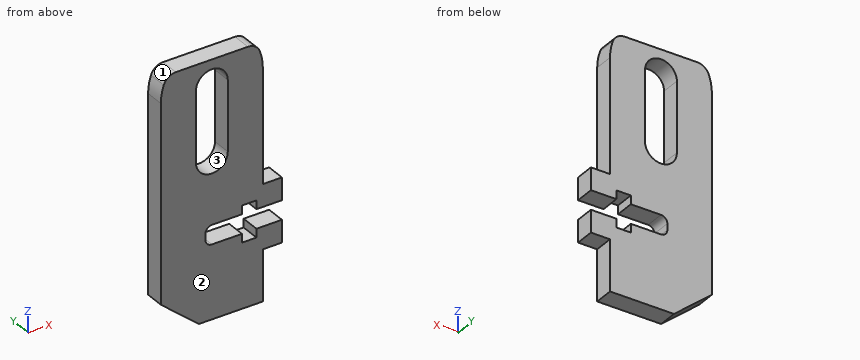
```python
from build123d import *

# Parameters (mm, degrees)
BOSS_EXTRUDE1_DEPTH     = 1.5
CUT_EXTRUDE1_DEPTH      = 38.54894195
CUT_EXTRUDE1_DEPTH_BACK = 38.54894195


with BuildPart() as part:
    # Sketch2 → Boss-Extrude1 (new, symmetric)
    with BuildSketch(Plane(origin=(0, 0, 0), x_dir=(1, 0, 0), z_dir=(0, 1, 0))):
        with BuildLine():
            Line((-8, 10.748624987), (-8, 30.870225))
            Line((-8, 30.870225), (-2.041232037, 35.870225))
            Line((-2.041232037, 35.870225), (8, 35.870225))
            Line((8, 35.870225), (8, 30.870225))
            Line((8, 30.870225), (8, 27.870225))
            Line((8, 27.870225), (11, 27.870225))
            Line((11, 27.870225), (11, 17.870225))
            Line((11, 17.870225), (8, 17.870225))
            Line((8, 17.870225), (8, 14.870225))
            Line((8, 14.870225), (8, 10.748624987))
            Line((8, 10.748624987), (8, 0))
            ThreePointArc((8, 0), (7.884788477, -1.35281583), (7.542472333, -2.666666667))
            ThreePointArc((7.542472333, -2.666666667), (6.811554788, -3.632993162), (5.656854249, -4))
            Line((5.656854249, -4), (-5.656854249, -4))
            ThreePointArc((-5.656854249, -4), (-6.811554788, -3.632993162), (-7.542472333, -2.666666667))
            ThreePointArc((-7.542472333, -2.666666667), (-7.884788477, -1.35281583), (-8, 0))
            Line((-8, 0), (-8, 10.748624987))
        make_face()
        with BuildLine():
            Line((-2.5, 0), (-2.5, 11))
            ThreePointArc((-2.5, 11), (0, 13.5), (2.5, 11))
            Line((2.5, 11), (2.5, 0))
            ThreePointArc((2.5, 0), (0, -2.5), (-2.5, 0))
        make_face(mode=Mode.SUBTRACT)
    extrude(amount=BOSS_EXTRUDE1_DEPTH, both=True)

    # Sketch4 → Cut-Extrude1 (cut, two sides: drawn at the far end of the back side and taken through both)
    with BuildSketch(Plane(origin=(0, 0, 0), x_dir=(1, 0, 0), z_dir=(0, 1, 0)).offset(-CUT_EXTRUDE1_DEPTH_BACK)):
        with BuildLine():
            Line((11, 24.370225), (7, 24.370225))
            Line((7, 24.370225), (7, 25.720225))
            Line((7, 25.720225), (4.73, 25.720225))
            Line((4.73, 25.720225), (4.73, 24.370225))
            Line((4.73, 24.370225), (0, 24.370225))
            ThreePointArc((0, 24.370225), (-0.707106781, 24.077331781), (-1, 23.370225))
            Line((-1, 23.370225), (-1, 22.370225))
            ThreePointArc((-1, 22.370225), (-0.707106781, 21.663118219), (0, 21.370225))
            Line((0, 21.370225), (4.73, 21.370225))
            Line((4.73, 21.370225), (4.73, 20.020225))
            Line((4.73, 20.020225), (7, 20.020225))
            Line((7, 20.020225), (7, 21.370225))
            Line((7, 21.370225), (11, 21.370225))
            Line((11, 21.370225), (11, 24.370225))
        make_face()
    extrude(amount=CUT_EXTRUDE1_DEPTH + CUT_EXTRUDE1_DEPTH_BACK, mode=Mode.SUBTRACT)


solid = part.part
```
The listing builds one solid part. Answer for the finished solid, in the listing's coordinates (mm). Face numbers are marked on the shaded views. Give positions to 0.01 mm unless a question says otherwise; leave off trailing zeros. Order: outer loops, then holes, each group sorted by start corner. A loop starts at its lowest first (then second) coordinate and runs counter-clockwise, first axis right, second up.
Item 1: Given pin 1 Ø1.5 at (x, y) = (9.5, -0.5) entering from +Z; pin 2 Ø0.9 at (y, z) = (0.5, -5) entering from +X; pin 3 Ø0.5 at (y, z) = (0.5, -23) entering from +X, each flat-ended and moving along its own axis, determine where each tip first touches the part or whether it passes through.
From the geometry:
pin 1: stops at z = -17.87
pin 2: stops at x = 8
pin 3: stops at x = -1
Item 2: Find the intervals of material crossed by probe 1 along X at (y, z) = (0.95, -11); probe 2 along Z at (x, y) = (5, -1.4); probe 3 along Z at (x, y) = (4.25, -0.95), in increasing order.
From the geometry:
probe 1: x = -8 to -2.5, 2.5 to 8
probe 2: z = -35.87 to -25.72, -20.02 to 4
probe 3: z = -35.87 to -24.37, -21.37 to 4
Item 3: The part is cut by section A-A, the plane x = 9.5. Give the vertices of the cut face in (y, z).
From the geometry:
outline: (-1.5, -27.87) - (1.5, -27.87) - (1.5, -24.37) - (-1.5, -24.37) - close; (-1.5, -21.37) - (1.5, -21.37) - (1.5, -17.87) - (-1.5, -17.87) - close
Item 4: The part is cut by section D-D, the plane x = 1.5. Give the vertices of the cut face in (y, z), and give its area (3 significant figures).
From the geometry:
outline: (-1.5, -35.87) - (1.5, -35.87) - (1.5, -24.37) - (-1.5, -24.37) - close; (-1.5, -21.37) - (1.5, -21.37) - (1.5, -13) - (-1.5, -13) - close; (-1.5, 2) - (1.5, 2) - (1.5, 4) - (-1.5, 4) - close
area: 65.6 mm2
Item 5: The part is cut by section B-B, the plane z = -4. Give the vertices of the cut face in (x, y), and give its area (3 significant figures).
From the geometry:
outline: (-8, -1.5) - (-2.5, -1.5) - (-2.5, 1.5) - (-8, 1.5) - close; (2.5, -1.5) - (8, -1.5) - (8, 1.5) - (2.5, 1.5) - close
area: 33.0 mm2
Item 6: For a pull along X with two mould halves and no side action, classify the marked faces 1, 2 and 3 as pulls with the +X half, pulls with the -X half, needs draft (parallel to the pull), parting line crosses it, or undercut.
From the geometry:
face 1: pulls with the -X half
face 2: needs draft
face 3: undercut
